from build123d import *

# Parameters (mm, degrees)
SKETCH1_R           = 4
SKETCH1_R_2         = 1
BOSS_EXTRUDE1_DEPTH = 6
SKETCH2_R           = 10.066838553
SKETCH2_R_2         = 3.5
CUT_EXTRUDE1_DEPTH  = 3
CHAMFER1_SIZE       = 1
SKETCH3_R           = 1
CUT_EXTRUDE2_DEPTH  = 9.246211251


with BuildPart() as part:
    # Sketch1 → Boss-Extrude1 (new, symmetric)
    with BuildSketch(Plane(origin=(0, 0, 0), x_dir=(1, 0, 0), z_dir=(0, 1, 0))):
        with Locations(Location((0, 0, 0), (0, 0, 270))):
            Circle(SKETCH1_R)
        with Locations(Location((0, 0, 0), (0, 0, 270))):
            Circle(SKETCH1_R_2, mode=Mode.SUBTRACT)
    extrude(amount=BOSS_EXTRUDE1_DEPTH, both=True)

    # Sketch2 → Cut-Extrude1 (cut, symmetric)
    with BuildSketch(Plane(origin=(0, 0, 0), x_dir=(1, 0, 0), z_dir=(0, 1, 0))):
        Circle(SKETCH2_R)
        with Locations(Location((0, 0, 0), (0, 0, 270))):
            Circle(SKETCH2_R_2, mode=Mode.SUBTRACT)
    extrude(amount=CUT_EXTRUDE1_DEPTH, both=True, mode=Mode.SUBTRACT)

    # Chamfer1
    # the kernel refuses this chamfer: 1 mm, written as the material it adds along each edge
    with BuildSketch(Plane(origin=(0, -3, 0), x_dir=(0, 0, 1), z_dir=(-1, 0, 0))) as chamfer1_piece_1_section:
        Polygon((3.5 + CHAMFER1_SIZE, 0), (3.5, CHAMFER1_SIZE), (3.5, 0), align=None)
    chamfer1_piece_1 = revolve(axis=Axis((0, -3, 0), (0, 1, 0)), mode=Mode.PRIVATE)
    chamfer1_piece_1 = chamfer1_piece_1 & Plane(origin=(0, -2.250849305, 0), x_dir=(0, 0, 1), z_dir=(0, 1, 0)) * Cylinder(4, 18, mode=Mode.PRIVATE)
    add(chamfer1_piece_1)
    with BuildSketch(Plane(origin=(0, 3, 0), x_dir=(0, 0, 1), z_dir=(-1, 0, 0))) as chamfer1_piece_2_section:
        Polygon((3.5, -CHAMFER1_SIZE), (3.5 + CHAMFER1_SIZE, 0), (3.5, 0), align=None)
    chamfer1_piece_2 = revolve(axis=Axis((0, 3, 0), (0, 1, 0)), mode=Mode.PRIVATE)
    chamfer1_piece_2 = chamfer1_piece_2 & Plane(origin=(0, 2.250849305, 0), x_dir=(0, 0, 1), z_dir=(0, 1, 0)) * Cylinder(4, 18, mode=Mode.PRIVATE)
    add(chamfer1_piece_2)

    # Sketch3 → Cut-Extrude2 (cut, through all)
    with BuildSketch(Plane.XY):
        with Locations(Location((0, 4.25, 0), (0, 0, 270))):
            Circle(SKETCH3_R)
        with Locations(Location((0, -4.25, 0), (0, 0, 270))):
            Circle(SKETCH3_R)
    extrude(amount=CUT_EXTRUDE2_DEPTH, mode=Mode.SUBTRACT)


solid = part.part
Part model, mm, in its own coordinate system. A direction names the side the tool comes from. Coordinates: 2 decimals unless noted, no trailing zeros. Write each loop counter-clockwise with the first axis right and the second up, starting at its lowest first coordinate (ties: lowest second). Pieces come first, ordered by that corner, then holes. Notation, with made-up numbers: (-30.5, 79) - (16.5, 79) arc R21 ccw to (16.5, 96) - close; hole circle Ø3 at (-16.5, 65). An arc over 180 degrees is marked (long way). Put each result on its own line as item: value.
1. Band-saw the part on A-A (x = 0). Write the cut outline in (y, z), then the cut area to 3 significant figures.
Final values:
outline: (-6, -4) - (-2.5, -4) - (-2, -3.5) - (2, -3.5) - (2.5, -4) - (6, -4) - (6, -1) - (-6, -1) - close; (-6, 1) - (-5.25, 1) - (-5.25, 4) - (-6, 4) - close; (-3.25, 1) - (3.25, 1) - (3.25, 4) - (2.5, 4) - (2, 3.5) - (-2, 3.5) - (-2.5, 4) - (-3.25, 4) - close; (5.25, 1) - (6, 1) - (6, 4) - (5.25, 4) - close
area: 55.5 mm²
2. Flat gauge pins, fed straight in: pin 1 Ø1.5 at (x, y) = (-1.5, 3) entering from -Z; pin 2 Ø1.5 at (x, y) = (-1, 0.5) entering from -Z; pin 3 Ø1 at (y, z) = (-3.5, 1) entering from +X; pin 4 Ø1.2 at (x, z) = (0, 0) entering from -Y. Where does each tip first touch, or does it go through?
Final values:
pin 1: stops at z = -3.93
pin 2: stops at z = -3.49
pin 3: stops at x = 3.97
pin 4: passes through
3. Band-saw the part on D-D (y = 1.5). Write the cut outline in (x, z), then the cut area to 3 significant figures.
Final values:
outline: circle Ø7 at (0, 0); hole circle Ø2 at (0, 0)
area: 35.3 mm²
4. Band-saw the part on B-B (y = 3). Write the cut outline in (x, z).
Final values:
outline: circle Ø8 at (0, 0); hole circle Ø2 at (0, 0)
5. Probe line 1 along Y through (x, z) = (0, 2.45); line 2 along X through (y, z) = (-0.5, 0); line 3 along X through (y, z) = (-2.75, 0). List the from-to ranges inside material, lowest first. Write a range as [from, to].
Final values:
line 1: y = [-6, -5.25], [-3.25, 3.25], [5.25, 6]
line 2: x = [-3.5, -1], [1, 3.5]
line 3: x = [-4, -1], [1, 4]
6. Band-saw the part on C-C (z = 2.75). Give the number of separate pieces and of enclosed holes in the cut face, then the cut area to 3 significant figures.
Final values:
separate pieces: 1
enclosed holes: 2
area: 56.8 mm²
7. Two-plate mould, pull along X, no slides. Class faces 4 (the cylindrical face through (0, 0, -1)), 5 (the cylindrical face through (-3.905, -4.226, -0.867)), 6 (the flat face through (-1, 6, 1)), 7 (the cylindrical face through (0.84, 3.71, 2.42)): +X half, -X half, draft (parallel to the pull), parting line (faces both ways), or undercut.
Final values:
face 4: undercut
face 5: parting line
face 6: draft
face 7: undercut
8. 3-axis set-ups, long thin cutter, end or side, ignore diameter. For faces 1 (the flat face through (-1, -6, 1)), 2 (the cylindrical face through (-3.417, -0.028, -0.759)), 3 (the cylindrical face through (0.84, -4.79, 2.42)): which of +Z, -Z, +X, -X, +Y, -Y reach the whole face in a straight line?
Final values:
face 1: +Z, -Z, +X, -X, -Y
face 2: none
face 3: +Z
